```python
from build123d import *

# Parameters (mm, degrees)
SKETCH_2_OUTSIDE_W   = 37.95
SKETCH_2_OUTSIDE_H   = 37.95
SKETCH_2_OUTSIDE_W_2 = 5.5
SKETCH_2_OUTSIDE_H_2 = 17
CUT_EXTRUDE_1_DEPTH  = 4.5
CHAMFER_3_SIZE       = 0.5


with BuildPart() as part:
    # Эскиз1 → Повернуть1 (revolve)
    with BuildSketch(Plane(origin=(0, 0, 0), x_dir=(1, 0, 0), z_dir=(0, 1, 0))):
        with BuildLine():
            Line((14, 0), (14, 1.276685932))
            ThreePointArc((14, 1.276685932), (7.087720463, 2.940710488), (0, 3.5))
            Line((0, 3.5), (0, 0))
            Line((0, 0), (14, 0))
        make_face()
    revolve(axis=Axis((0, 0, -3.5), (0, 0, 1)))

    # Эскиз2 outside → Вырез-Вытянуть1 (cut, through all)
    with BuildSketch(Plane.XY):
        Rectangle(SKETCH_2_OUTSIDE_W, SKETCH_2_OUTSIDE_H)
        with Locations((-4.05, 3.7)):
            Rectangle(SKETCH_2_OUTSIDE_W_2, SKETCH_2_OUTSIDE_H_2, mode=Mode.SUBTRACT)
    extrude(amount=-CUT_EXTRUDE_1_DEPTH, mode=Mode.SUBTRACT)

    # Фаска3
    chamfer_3_edges = [part.edges().sort_by_distance(p)[0] for p in [
        (-1.3, -4.8, -1.61277204),
    ]]
    chamfer(chamfer_3_edges, length=CHAMFER_3_SIZE)


solid = part.part
```
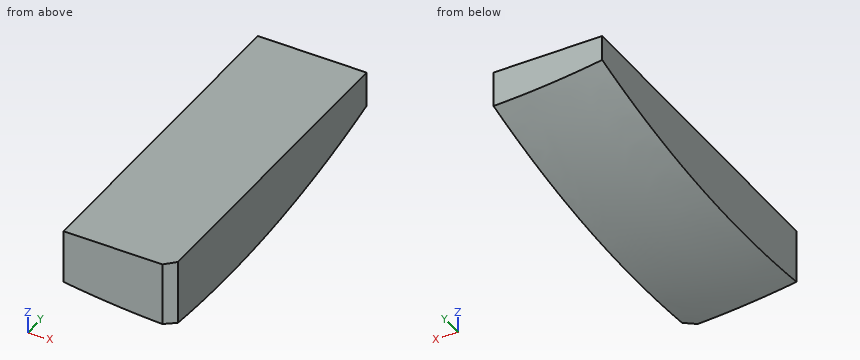
The listing builds one solid part. Answer for the finished solid, in the listing's coordinates (mm). Give positions to 0.01 mm unless a question says otherwise; leave off trailing zeros. Order: outer loops, then holes, each group sorted by start corner. A loop starts at its lowest first (then second) coordinate and runs counter-clockwise, first axis right, second up. Notation, with made-up numbers: (-7, 81.5) -> (8, 81.5) arc R24 cw to (8, 97.5) -> close; hole circle Ø8 at (-39.75, 27.5). An arc over 180 degrees is marked (long way). Answer as CSV lines item,"result". Start each with the question number.
Q1. A cutting plane is placed at B-B (z = -1.65). Determine the outline of the cut face in (x, y).
Q2. A cutting plane is placed at C-C (x = -6.15). Determine the outline of the cut face in (y, z).
Q3. Given pin 1 (1 mm diameter, centred on x = -5.5, y = 9.5, fed in from -Z), flat-ended and moving along its own axis, determine where the tip first touches the part or whether it passes through.
Q4. Find the intervals of material crossed by L1, parallel to Z at x = -5.15, y = 7.25; L2, parallel to Z at x = -5.85, y = 9, in increasing order.
Q5. A cutting plane is placed at D-D (z = -2.3). Determine the outline of the cut face in (x, y), then the cut area to 3 significant figures.
Q6. A cutting plane is placed at A-A (y = 0). Determine the outline of the cut face in (x, z), then the cut area to 3 significant figures.
Results found:
1,outline,"(-6.8, -4.8) -> (-1.8, -4.8) -> (-1.3, -4.3) -> (-1.3, 12.2) -> (-3.87, 12.2) arc R12.8 ccw to (-6.8, 10.84) -> close"
2,outline,"(-4.8, -2.82) arc R44.77 ccw to (12.2, -1.39) -> (12.2, 0) -> (-4.8, 0) -> close"
3,pin 1,"z = -2.27"
4,L1,"-2.62 to 0"
4,L2,"-2.21 to 0"
5,outline,"(-6.8, -4.8) -> (-1.8, -4.8) -> (-1.3, -4.3) -> (-1.3, 10.26) arc R10.34 ccw to (-6.8, 7.8) -> close"
5,area,"77.7 mm2"
6,outline,"(-6.8, -2.99) arc R45.19 ccw to (-1.3, -3.48) -> (-1.3, 0) -> (-6.8, 0) -> close"
6,area,"18.1 mm2"
